from build123d import *

# Parameters (mm, degrees)
F3_W     = 24.3006017764
F3_H     = 12.100000065
F3_R     = 1
F4_DEPTH = 3


# Not quite as in the source:
# - ends of sketch curves that miss each other by under 0.0002 mm in the source are joined


with BuildPart() as f4:
    # F3 (on Front) → F4 (new body)
    with BuildSketch(Plane.XZ):
        Polygon((-18.3427034128, 0), (-17.3427034128, 0), (-17.3423305717, 1.9999998262), (-18.1417713099, 1.9999998262), (-18.1417713099, 4.9999998262), (-17.3417713099, 4.9999998262), (-17.3415848893, 5.9999998262), (-16.3415848684, 5.9999998262), (-16.3417712925, 4.9999998262), (-15.5417712925, 4.9999998262), (-15.5417712925, 1.9999998262), (-16.3423305647, 1.9999998262), (-16.3427034128, 0), (-15.3427034128, 0), (-6.8427034128, 0), (8.1310835591, 0), (8.1572965872, 0), (16.6572965872, 0), (17.7038592511, 0), (17.704234553, 2.0131421474), (16.9047938148, 2.0131421517), (16.9047938308, 5.0131421517), (17.7047938308, 5.0131421475), (17.7049802567, 6.0131421474), (18.7049802776, 6.0131421421), (18.7047938482, 5.0131421421), (19.5047938482, 5.0131421378), (19.5047938321, 2.0131421378), (18.7042345599, 2.0131421421), (18.703859251, 0), (19.6572965872, 0), (23.5180836171, 0), (23.5180836171, 30), (18.7038593313, 30), (18.7042346294, 27.9868579887), (19.5047939016, 27.9868579887), (19.5047939016, 24.9868579887), (18.7047939016, 24.9868579887), (18.7049803257, 23.9868579887), (17.7049803048, 23.9868579887), (17.7047938842, 24.9868579887), (16.9047938842, 24.9868579887), (16.9047938842, 27.9868579887), (17.7042346225, 27.9868579887), (17.7038593313, 30), (8.0515714362, 30), (0, 30), (-7.0037143305, 30), (-16.3427034128, 30), (-16.3423305647, 28.0000001738), (-15.5417712925, 28.0000001738), (-15.5417712925, 25.0000001738), (-16.3417712925, 25.0000001738), (-16.3415848684, 24.0000001738), (-17.3415848893, 24.0000001738), (-17.3417713099, 25.0000001738), (-18.1417713099, 25.0000001738), (-18.1417713099, 28.0000001738), (-17.3423305717, 28.0000001738), (-17.3427034128, 30), (-21.7979144805, 30), (-21.7979144805, 28.0000001738), (-21.7979144805, 25.0000001738), (-21.7979144805, 24.0000001738), (-21.7979144805, 15.0000001738), (-21.7979144805, 1.738e-07), align=None)
        with BuildLine():
            ThreePointArc((-19.593004301, 15.0000001705), (-20.5930043024, 14.0000001705), (-21.593004301, 15.0000001732))
            ThreePointArc((-21.593004301, 15.0000001732), (-20.5930042997, 16.0000001705), (-19.593004301, 15.0000001705))
        make_face(mode=Mode.SUBTRACT)
        with Locations((-6.593004301, 15.0000001331)):
            Rectangle(F3_W, F3_H, mode=Mode.SUBTRACT)
        with Locations((7.406995699, 15.0000000956)):
            Circle(F3_R, mode=Mode.SUBTRACT)
        Polygon((-7.0037143305, 33), (-7.0037143305, 30), (0, 30), (8.0515714362, 30), (8.0409989211, 33), align=None)
        Polygon((8.1310835591, 0), (-6.8427034128, 0), (-6.826602321, -3), (0, -3), (8.1678691023, -3), (8.1572965872, 0), align=None)
    extrude(amount=F4_DEPTH)


solid = f4.part
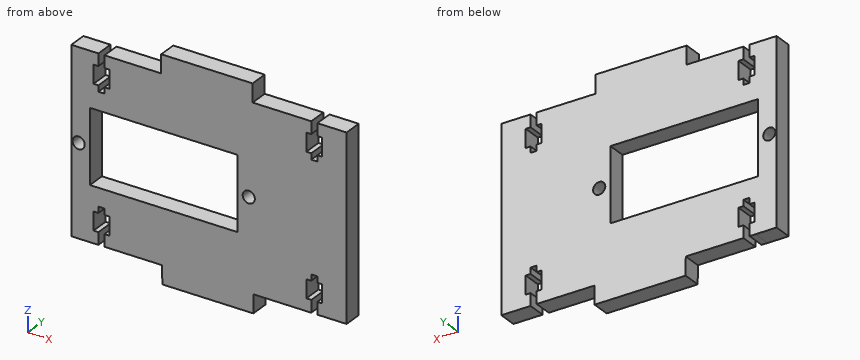
For this review, take the finished solid that the model builds, in its own axes (mm). Give positions to 0.01 mm unless a question says otherwise; leave off trailing zeros. Order: outer loops, then holes, each group sorted by start corner. A loop starts at its lowest first (then second) coordinate and runs counter-clockwise, first axis right, second up. Notation, with made-up numbers: M -36.5,39 L -29.5,39 A9 cw -29.5,50 Z; hole C 73,0 d3. An arc over 180 degrees is marked long. Answer in a Markdown table with one row per item. Add a question column.
(1) Consider section A-A on z = 17. State the section outline as (x, y) points, and give its area (3 significant figures).
(2) Consider section D-D on x = 13. State the section outline as (y, z) points, and give its area (3 significant figures).
(3) For pin 1 (0.9 mm diameter, centred on x = -12.5, y = -1, fed in from -Z), flat-tipped, find the tip position at first contact; note if it passes through.
(4) Consider section B-B on z = 3. State the section outline as (x, y) points, and give its area (3 significant figures).
(5) Consider section C-C on x = -2. State the section outline as (y, z) points.
(6) Wall thickness on probe 1 along Z at (x, y) = (19, -1.4); probe 2 along X at (y, z) = (-0.8, 29); probe 3 along Z at (x, y) = (-4, -1.45): over which ranges is each line inside the solid? List them lowest first. Write a range as [from, to].
Evaluation:
| question | item | result |
|---|---|---|
| 1 | outline | M -21.8,-3 L -18.74,-3 L -18.74,0 L -21.8,0 Z; M 5.56,-3 L 23.52,-3 L 23.52,0 L 5.56,0 Z |
| 1 | area | 63.0 mm^2 |
| 2 | outline | M -3,0 L 0,0 L 0,30 L -3,30 Z |
| 2 | area | 90.0 mm^2 |
| 3 | pin 1 | stops at z = 0 |
| 4 | outline | M -21.8,-3 L -18.14,-3 L -18.14,0 L -21.8,0 Z; M -15.54,-3 L 16.9,-3 L 16.9,0 L -15.54,0 Z; M 19.5,-3 L 23.52,-3 L 23.52,0 L 19.5,0 Z |
| 4 | area | 120 mm^2 |
| 5 | outline | M -3,-3 L 0,-3 L 0,8.95 L -3,8.95 Z; M -3,21.05 L 0,21.05 L 0,33 L -3,33 Z |
| 6 | probe 1 | z = [0, 2.01], [5.01, 24.99], [27.99, 30] |
| 6 | probe 2 | x = [-21.8, -17.34], [-16.34, 17.7], [18.7, 23.52] |
| 6 | probe 3 | z = [-3, 8.95], [21.05, 33] |
